Read the model definition and answer for the solid it produces. Units are mm, in the model's axes. A direction names the side the tool comes from. Give positions to 0.01 mm unless a question says otherwise; leave off trailing zeros. Order: outer loops, then holes, each group sorted by start corner. A loop starts at its lowest first (then second) coordinate and runs counter-clockwise, first axis right, second up.
Item 1: A cutting plane is placed at C-C (x = -132.75). Write down the section's boundary in (y, z).
Item 2: Given pin 1 Ø10 at (x, z) = (75.5, 5.5) entering from +Y; pin 2 Ø4.5 at (y, z) = (-18.5, 19) entering from +X; pin 3 Ø4.5 at (y, z) = (-42.5, 17) entering from -X, each flat-ended and moving along its own axis, determine where each tip first touches the part or whether it passes through.
Item 3: The mould has two halves that part along X. Classify faces 4 (the face through (-10, -33, 18)), 5 (the face through (-10.4, -40.5, 10)), 6 (the face through (135.06, 33.27, 18.46)), 7 (the face through (-12.5, -33, 18)): +X half, -X half, draft (parallel to the pull), parting line (faces both ways), or undercut.
Item 4: Which of the six approach directions +Z, -Z, +X, -X, +Y, -Y give full straight-line access (tool end or side, diameter ignored) to faces 1 (the face through (-117.5, 17, 17)), 2 (the face through (120, 15, 17)), 3 (the face through (-10.4, -40.5, 25))?
Item 5: A cutting plane is placed at A-A (y = 28). Write down the section's boundary in (x, z), plus the area to 3 significant figures.
Item 6: Find the intervals of material crossed by line 1 along X through (y, z) = (32.65, 17.5); line 2 along X through (y, z) = (27, 21.5); line 3 along Z through (x, y) = (-132.75, 33.9), in increasing order.
Item 7: A cutting plane is placed at B-B (z = 17.5). State how many separate pieces and enclosed holes the cut face has, plus the area to 3 significant figures.
from build123d import *

# Parameters (mm, degrees)
BOSS_EXTRUDE1_DEPTH = 35
SKETCH2_R           = 2.5
SKETCH2_W           = 32
SKETCH2_H           = 20
CUT_EXTRUDE1_DEPTH  = 90
BOSS_EXTRUDE2_DEPTH = 7.5


with BuildPart() as part:
    # Sketch1 → Boss-Extrude1 (new body)
    with BuildSketch(Plane.XY):
        Polygon((117.5, 0), (-117.5, 0), (-117.5, 34.5), (-142.5, 34.5), (-142.5, 32), (-120, 32), (-120, -2.5), (120, -2.5), (120, 32), (142.5, 32), (142.5, 34.5), (117.5, 34.5), align=None)
    extrude(amount=BOSS_EXTRUDE1_DEPTH)

    # Sketch2 → Cut-Extrude1 (cut)
    with BuildSketch(Plane(origin=(0, 34.5, 0), x_dir=(1, 0, 0), z_dir=(0, 1, 0))):
        with Locations((-132.75, -17.5)):
            Circle(SKETCH2_R)
        with Locations((132.75, -17.5)):
            Circle(SKETCH2_R)
        with Locations((7.8, -17.5)):
            Rectangle(SKETCH2_W, SKETCH2_H)
    extrude(amount=-CUT_EXTRUDE1_DEPTH, mode=Mode.SUBTRACT)

    # Sketch4 → Boss-Extrude2 (add, symmetric)
    with BuildSketch(Plane.XY.offset(17.5)):
        Polygon((-12.5, -2.5), (-12.5, -65), (27.5, -65), (27.5, -2.5), (25, -2.5), (25, -62.5), (-10, -62.5), (-10, -2.5), align=None)
    extrude(amount=BOSS_EXTRUDE2_DEPTH, both=True)


solid = part.part
Response values:
1. outline: (32, 0) - (34.5, 0) - (34.5, 15) - (32, 15) - close; (32, 20) - (34.5, 20) - (34.5, 35) - (32, 35) - close
2. pin 1: stops at y = 0
2. pin 2: stops at x = 27.5
2. pin 3: stops at x = -12.5
3. face 4: undercut
3. face 5: draft
3. face 6: undercut
3. face 7: -X half
4. face 1: +Z, -Z, +Y
4. face 2: +Z, -Z, +X, -Y
4. face 3: +Z, +X, -X, -Y
5. outline: (-120, 0) - (-117.5, 0) - (-117.5, 35) - (-120, 35) - close; (117.5, 0) - (120, 0) - (120, 35) - (117.5, 35) - close
5. area: 175 mm2
6. line 1: x = -142.5 to -135.25, -130.25 to -117.5, 117.5 to 130.25, 135.25 to 142.5
6. line 2: x = -120 to -117.5, 117.5 to 120
6. line 3: z = 0 to 15, 20 to 35
7. separate pieces: 3
7. enclosed holes: 0
7. area: 1,180 mm2
